Source: three-view drawing plus pictorial views. Frame: mm from the lowest corner of the part. Give positions to 0.01 mm unless a question says otherwise; leave off trailing zeros. Order: outer loops, then holes, each group sorted by start corner. A loop starts at its lowest first (then second) coordinate and runs counter-clockwise, first axis right, second up.
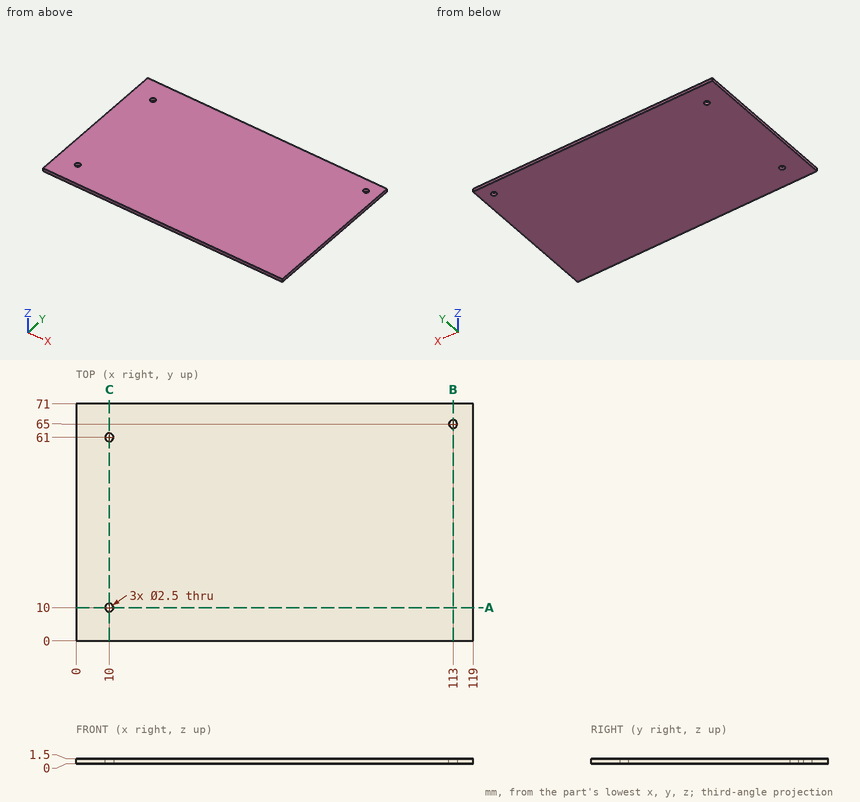
(1) Line query: line 1 along Y through (x, z) = (113, 0.65); line 2 along X through (y, z) = (65, 0.95); line 3 along X through (y, z) = (61.5, 1.15). Output: solid intervals per line, ascending.
(2) Section A-A, the plane y = 10. Return loops of the section in (x, z).
(3) Pin query (flat end, axial travel): pin 1 Ø2 at (x, y) = (113, 65) entering from +Z. Return the tip coordinate at first contact, or that it passes through.
(4) Section C-C, the plane x = 10. Return loops of the section in (y, z), plus the area to 3 significant figures.
(5) Section B-B, the plane x = 113. Return loops of the section in (y, z), plus the area to 3 significant figures.
Checks:
1. line 1: y = 0 to 63.75, 66.25 to 71
1. line 2: x = 0 to 111.75, 114.25 to 119
1. line 3: x = 0 to 8.85, 11.15 to 119
2. outline: (0, 0) - (8.75, 0) - (8.75, 1.5) - (0, 1.5) - close; (11.25, 0) - (119, 0) - (119, 1.5) - (11.25, 1.5) - close
3. pin 1: passes through
4. outline: (0, 0) - (8.75, 0) - (8.75, 1.5) - (0, 1.5) - close; (11.25, 0) - (59.75, 0) - (59.75, 1.5) - (11.25, 1.5) - close; (62.25, 0) - (71, 0) - (71, 1.5) - (62.25, 1.5) - close
4. area: 99.0 mm2
5. outline: (0, 0) - (63.75, 0) - (63.75, 1.5) - (0, 1.5) - close; (66.25, 0) - (71, 0) - (71, 1.5) - (66.25, 1.5) - close
5. area: 103 mm2
